```python
from build123d import *

# Parameters (mm, degrees)
BOSS_EXTRUDE1_DEPTH = 7.62
SKETCH2_R           = 1.905
CUT_EXTRUDE1_DEPTH  = 5.08


with BuildPart() as part:
    # Sketch1 → Boss-Extrude1 (new body)
    with BuildSketch(Plane.XY):
        with BuildLine():
            Line((1.905, 6.985), (-1.905, 6.985))
            ThreePointArc((-1.905, 6.985), (-2.301749521, 6.845797154), (-2.524550498, 6.489219898))
            ThreePointArc((-2.524550498, 6.489219898), (-3.583781011, 3.443081012), (-5.301992306, 0.713853771))
            ThreePointArc((-5.301992306, 0.713853771), (-5.964076777, 0.187711648), (-6.788664987, 0))
            Line((-6.788664987, 0), (-12.985936717, 0))
            Line((-12.985936717, 0), (-12.985936717, 1.073162668))
            ThreePointArc((-12.985936717, 1.073162668), (-12.799949523, 1.522175474), (-12.350936717, 1.708162668))
            Line((-12.350936717, 1.708162668), (-6.788664987, 1.708162668))
            ThreePointArc((-6.788664987, 1.708162668), (-6.488026831, 1.77904797), (-6.250721894, 1.976770993))
            ThreePointArc((-6.250721894, 1.976770993), (-4.890441533, 4.244637177), (-4.029326465, 6.745049248))
            ThreePointArc((-4.029326465, 6.745049248), (-3.010501923, 8.43943232), (-1.085423689, 8.89))
            Line((-1.085423689, 8.89), (1.085423689, 8.89))
            ThreePointArc((1.085423689, 8.89), (3.010501923, 8.43943232), (4.029326465, 6.745049248))
            ThreePointArc((4.029326465, 6.745049248), (4.890441533, 4.244637177), (6.250721894, 1.976770993))
            ThreePointArc((6.250721894, 1.976770993), (6.488026831, 1.77904797), (6.788664987, 1.708162668))
            Line((6.788664987, 1.708162668), (12.350936717, 1.708162668))
            ThreePointArc((12.350936717, 1.708162668), (12.799949523, 1.522175474), (12.985936717, 1.073162668))
            Line((12.985936717, 1.073162668), (12.985936717, 0))
            Line((12.985936717, 0), (6.788664987, 0))
            ThreePointArc((6.788664987, 0), (5.964076777, 0.187711648), (5.301992306, 0.713853771))
            ThreePointArc((5.301992306, 0.713853771), (3.583781011, 3.443081012), (2.524550498, 6.489219898))
            ThreePointArc((2.524550498, 6.489219898), (2.301749521, 6.845797154), (1.905, 6.985))
        make_face()
    extrude(amount=BOSS_EXTRUDE1_DEPTH)

    # Sketch2 → Cut-Extrude1 (cut)
    with BuildSketch(Plane(origin=(0, 1.708162668, 0), x_dir=(1, 0, 0), z_dir=(0, 1, 0))):
        with Locations(Location((9.525, -3.81, 0), (0, 0, 270))):
            Circle(SKETCH2_R)
        with Locations(Location((-9.525, -3.81, 0), (0, 0, 270))):
            Circle(SKETCH2_R)
    extrude(amount=-CUT_EXTRUDE1_DEPTH, mode=Mode.SUBTRACT)


solid = part.part
```
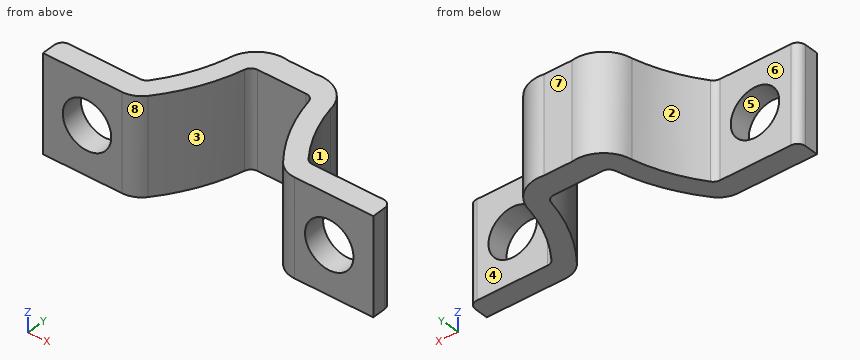
The listing builds one solid part. Answer for the finished solid, in the listing's coordinates (mm). Face numbers are marked on the shaded views. A direction names the side the tool comes from. Coordinates: 2 decimals unless noted, no trailing zeros. Write each loop counter-clockwise with the first axis right and the second up, starting at its lowest first coordinate (ties: lowest second). Pieces come first, ordered by that corner, then holes. Notation, with made-up numbers: (11.5, 30) -> (16.5, 30) arc R25 cw to (16.5, 50) -> close; hole circle Ø10 at (0.25, -1.75). An arc over 180 degrees is marked (long way). Write each question's results on one line, items separated by ' | '. Start each with the question number.
1) A cutting plane is placed at A-A (x = 10.75). Determine the outline of the cut face in (y, z), then the cut area to 3 significant figures.
2) A cutting plane is placed at C-C (y = 5.75). Determine the outline of the cut face in (x, z).
3) A cutting plane is placed at D-D (z = 6.5). Determine the outline of the cut face in (x, y) (3 decimals).
4) Straight lines are drawn through the part: probe 1 along X at (y, z) = (0.85, 3.81); probe 2 along Y at (x, z) = (-0.25, 0.5) (3 decimals); probe 3 along X at (y, z) = (0.4, 3.81). For each, find the intervals that lie inside material, in ascending order.
5) A cutting plane is placed at B-B (z = 3.81). Count the separate pieces of the cut face and the enclosed holes in it, then the cut area to 3 significant figures.
6) For a pull along X with two mould halves and no side action, classify the marked faces 1, 2, 3 and 4 as +X half, -X half, draft (parallel to the pull), parting line (faces both ways), or undercut.
7) Flat-ended cylindrical pins translate along their axes: pin 1 Ø4.5 at (x, z) = (9.525, 3.81) entering from +Y; pin 2 Ø1 at (y, z) = (7.5, 5) entering from +X; pin 3 Ø1.7 at (x, z) = (0.5, 3.5) entering from +Y. Find the tip coordinate at first contact, or state that the pin passes through.
8) A tool of negligible diameter and unlimited length cuts with its end or side. For the marked faces 5, 6, 7 and 8, from which of +Z, -Z, +X, -X, +Y, -Y can it reach the whole face along a straight path? Write none if from no direction.
Values follow:
1) outline: (0, 0) -> (1.71, 0) -> (1.71, 2.35) -> (0, 2.35) -> close; (0, 5.27) -> (1.71, 5.27) -> (1.71, 7.62) -> (0, 7.62) -> close | area: 8.03 mm²
2) outline: (-4.3, 0) -> (-2.71, 0) -> (-2.71, 7.62) -> (-4.3, 7.62) -> close; (2.71, 0) -> (4.3, 0) -> (4.3, 7.62) -> (2.71, 7.62) -> close
3) outline: (-12.986, 0) -> (-6.789, 0) arc R1.905 ccw to (-5.302, 0.714) arc R14.224 ccw to (-2.525, 6.489) arc R0.635 cw to (-1.905, 6.985) -> (1.905, 6.985) arc R0.635 cw to (2.525, 6.489) arc R14.224 ccw to (5.302, 0.714) arc R1.905 ccw to (6.789, 0) -> (12.986, 0) -> (12.986, 1.073) arc R0.635 ccw to (12.351, 1.708) -> (6.789, 1.708) arc R0.673 cw to (6.251, 1.977) arc R12.7 cw to (4.029, 6.745) arc R2.54 ccw to (1.085, 8.89) -> (-1.085, 8.89) arc R2.54 ccw to (-4.029, 6.745) arc R12.7 cw to (-6.251, 1.977) arc R0.673 cw to (-6.789, 1.708) -> (-12.351, 1.708) arc R0.635 ccw to (-12.986, 1.073) -> close
4) probe 1: -12.99 to -11.43, -7.62 to -5.19, 5.19 to 7.62, 11.43 to 12.99 | probe 2: 6.985 to 8.89 | probe 3: -12.99 to -11.43, -7.62 to -5.62, 5.62 to 7.62, 11.43 to 12.99
5) separate pieces: 3 | enclosed holes: 0 | area: 43.9 mm²
6) face 1: +X half | face 2: -X half | face 3: undercut | face 4: draft
7) pin 1: y = 1.71 | pin 2: x = 3.98 | pin 3: y = 8.92
8) face 5: +Y, -Y | face 6: +Z, -Z, -X, +Y | face 7: +Z, -Z, +Y | face 8: +Z, -Z, -Y
